```python
from build123d import *

# Parameters (mm, degrees)
SKETCH_1_R      = 1.6
SKETCH_1_W      = 90
SKETCH_1_H      = 46.291651246
EXTRUDE_1_DEPTH = 3
FILLET_1_R      = 1
FILLET_2_R      = 10


with BuildPart() as part:
    # ｽｹｯﾁ1 → ﾎﾞｽ - 押し出し1 (new body)
    with BuildSketch(Plane.XY):
        with BuildLine():
            Line((50, 33.145825623), (-50, 33.145825623))
            ThreePointArc((-50, 33.145825623), (-52.5, 32.475952642), (-54.330127019, 30.645825623))
            Line((-54.330127019, 30.645825623), (-86.830127019, -25.645825623))
            ThreePointArc((-86.830127019, -25.645825623), (-86.830127019, -30.645825623), (-82.5, -33.145825623))
            Line((-82.5, -33.145825623), (-50, -33.145825623))
            Line((-50, -33.145825623), (50, -33.145825623))
            Line((50, -33.145825623), (82.5, -33.145825623))
            ThreePointArc((82.5, -33.145825623), (86.830127019, -30.645825623), (86.830127019, -25.645825623))
            Line((86.830127019, -25.645825623), (54.330127019, 30.645825623))
            ThreePointArc((54.330127019, 30.645825623), (52.5, 32.475952642), (50, 33.145825623))
        make_face()
        with Locations((-50, 28.145825623)):
            Circle(SKETCH_1_R, mode=Mode.SUBTRACT)
        with Locations((-82.5, -28.145825623)):
            Circle(SKETCH_1_R, mode=Mode.SUBTRACT)
        with Locations((50, 28.145825623)):
            Circle(SKETCH_1_R, mode=Mode.SUBTRACT)
        with Locations((82.5, -28.145825623)):
            Circle(SKETCH_1_R, mode=Mode.SUBTRACT)
        with Locations((-50, -28.145825623)):
            Circle(SKETCH_1_R, mode=Mode.SUBTRACT)
        with Locations((50, -28.145825623)):
            Circle(SKETCH_1_R, mode=Mode.SUBTRACT)
        with Locations((-35, -28.145825623)):
            Circle(SKETCH_1_R, mode=Mode.SUBTRACT)
        with Locations(Location((35, -28.145825623, 0), (0, 0, 180))):
            Circle(SKETCH_1_R, mode=Mode.SUBTRACT)
        with Locations((-15, 28.145825623)):
            Circle(SKETCH_1_R, mode=Mode.SUBTRACT)
        with Locations(Location((15, 28.145825623, 0), (0, 0, 180))):
            Circle(SKETCH_1_R, mode=Mode.SUBTRACT)
        with Locations((-50, -8.145825623)):
            Circle(SKETCH_1_R, mode=Mode.SUBTRACT)
        with Locations(Location((50, -8.145825623, 0), (0, 0, 180))):
            Circle(SKETCH_1_R, mode=Mode.SUBTRACT)
        Rectangle(SKETCH_1_W, SKETCH_1_H, mode=Mode.SUBTRACT)
        with BuildLine():
            Line((-55, 19.485571585), (-55, -28.145825623))
            Line((-55, -28.145825623), (-77.5, -28.145825623))
            ThreePointArc((-77.5, -28.145825623), (-78.169872981, -25.645825623), (-80, -23.815698604))
            Line((-80, -23.815698604), (-55, 19.485571585))
        make_face(mode=Mode.SUBTRACT)
        with BuildLine():
            Line((55, -28.145825623), (77.5, -28.145825623))
            ThreePointArc((77.5, -28.145825623), (78.169872981, -25.645825623), (80, -23.815698604))
            Line((80, -23.815698604), (55, 19.485571585))
            Line((55, 19.485571585), (55, -28.145825623))
        make_face(mode=Mode.SUBTRACT)
    extrude(amount=EXTRUDE_1_DEPTH)

    # ﾌｨﾚｯﾄ1
    fillet_1_edges = [part.edges().sort_by_distance(p)[0] for p in [
        (-55, 19.485571585, 1.5),
        (-80, -23.815698604, 1.5),
        (-77.5, -28.145825623, 1.5),
        (-55, -28.145825623, 1.5),
        (77.5, -28.145825623, 1.5),
        (80, -23.815698604, 1.5),
        (55, 19.485571585, 1.5),
        (55, -28.145825623, 1.5),
    ]]
    fillet(fillet_1_edges, radius=FILLET_1_R)

    # ﾌｨﾚｯﾄ2
    fillet_2_edges = [part.edges().sort_by_distance(p)[0] for p in [
        (45, -23.145825623, 1.5),
        (45, 23.145825623, 1.5),
        (-45, 23.145825623, 1.5),
        (-45, -23.145825623, 1.5),
    ]]
    fillet(fillet_2_edges, radius=FILLET_2_R)


solid = part.part
```
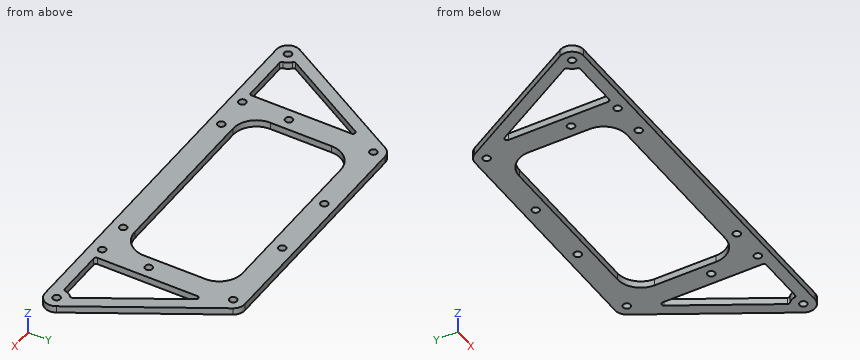
Part model, mm, in its own coordinate system. Coordinates: 2 decimals unless noted, no trailing zeros. Order: outer loops, then holes, each group sorted by start corner. A loop starts at its lowest first (then second) coordinate and runs counter-clockwise, first axis right, second up. Notation, with made-up numbers: (77.25, -16.5) - (87.25, -16.5) arc R20 ccw to (87.25, 5.5) - close; hole circle Ø9 at (78.5, -20.75). An arc over 180 degrees is marked (long way). Return JSON: item names as keys, results as strings. Group by question number.
Item 1: Cut at B-B (x = -9). List the corners of the cut face in (y, z), plus the area to 3 significant figures.
Item 2: Cut at C-C (y = 8). List the corners of the cut face in (x, z), plus the area to 3 significant figures.
Item 3: Cut at D-D (x = 62.5). List the corners of the cut face in (y, z).
Item 4: Drill centre lines: probe 1 along Y at (x, z) = (50, 2.15); probe 2 along Y at (x, z) = (-15, 2.15); probe 3 along Y at (x, z) = (-35, 2.3). Where is each one in solid material? Low to high. Write a range as from..to.
Item 5: Pin check, flat tips, straight feed: pin 1 (0.9 mm diameter, centred on y = -5.5, z = 2, fed in from -X); pin 2 (1 mm diameter, centred on y = 15, z = 1, fed in from +X); pin 3 (4 mm diameter, centred on x = 15, y = 28.15, fed in from +Z); pin 4 (1.5 mm diameter, centred on y = 17, z = 2.5, fed in from +X). Stop position of each tip, or through.
Item 6: Cut at A-A (x = 15). List the corners of the cut face in (y, z), plus the area to 3 significant figures.
Check values:
{
 "1": {"outline": "(-33.15, 0) - (-23.15, 0) - (-23.15, 3) - (-33.15, 3) - close; (23.15, 0) - (33.15, 0) - (33.15, 3) - (23.15, 3) - close", "area": "60.0 mm2"},
 "2": {"outline": "(-67.4, 0) - (-61.63, 0) - (-61.63, 3) - (-67.4, 3) - close; (-55, 0) - (-45, 0) - (-45, 3) - (-55, 3) - close; (45, 0) - (55, 0) - (55, 3) - (45, 3) - close; (61.63, 0) - (67.4, 0) - (67.4, 3) - (61.63, 3) - close", "area": "94.6 mm2"},
 "3": {"outline": "(-33.15, 0) - (-28.15, 0) - (-28.15, 3) - (-33.15, 3) - close; (6.5, 0) - (16.5, 0) - (16.5, 3) - (6.5, 3) - close"},
 "4": {"probe 1": "y = -33.15..-29.75, -26.55..-9.75, -6.55..26.55, 29.75..33.15", "probe 2": "y = -33.15..-23.15, 23.15..26.55, 29.75..33.15", "probe 3": "y = -33.15..-29.75, -26.55..-23.15, 23.15..33.15"},
 "5": {"pin 1": "stops at x = -75.46", "pin 2": "stops at x = 63.65", "pin 3": "stops at z = 3", "pin 4": "stops at x = 62.64"},
 "6": {"outline": "(-33.15, 0) - (-23.15, 0) - (-23.15, 3) - (-33.15, 3) - close; (23.15, 0) - (26.55, 0) - (26.55, 3) - (23.15, 3) - close; (29.75, 0) - (33.15, 0) - (33.15, 3) - (29.75, 3) - close", "area": "50.4 mm2"}
}
